from build123d import *

# Parameters (mm, degrees)
ESQUISSE1_R             = 15
BOSS_EXTRU_1_DEPTH      = 10
ESQUISSE2_R             = 12.5
BOSS_EXTRU_2_DEPTH      = 1
ESQUISSE3_R             = 11
ENL_V_MAT_EXTRU_1_DEPTH = 2
ESQUISSE4_R             = 12.5
ENL_V_MAT_EXTRU_2_DEPTH = 9


with BuildPart() as part:
    # Esquisse1 → Boss.-Extru.1 (new body)
    with BuildSketch(Plane.XY):
        Circle(ESQUISSE1_R)
    extrude(amount=BOSS_EXTRU_1_DEPTH)

    # Esquisse2 → Boss.-Extru.2 (add)
    with BuildSketch(Plane.XY.offset(10)):
        Circle(ESQUISSE2_R)
    extrude(amount=BOSS_EXTRU_2_DEPTH)

    # Esquisse3 → Enlèv. mat.-Extru.1 (cut)
    with BuildSketch(Plane.XY.offset(11)):
        Circle(ESQUISSE3_R)
    extrude(amount=-ENL_V_MAT_EXTRU_1_DEPTH, mode=Mode.SUBTRACT)

    # Esquisse4 → Enlèv. mat.-Extru.2 (cut)
    with BuildSketch(Plane(origin=(0, 0, 0), x_dir=(-1, 0, 0), z_dir=(0, 0, -1))):
        with Locations(Location((0, 0, 0), (0, 0, 180))):
            Circle(ESQUISSE4_R)
    extrude(amount=-ENL_V_MAT_EXTRU_2_DEPTH, mode=Mode.SUBTRACT)


solid = part.part
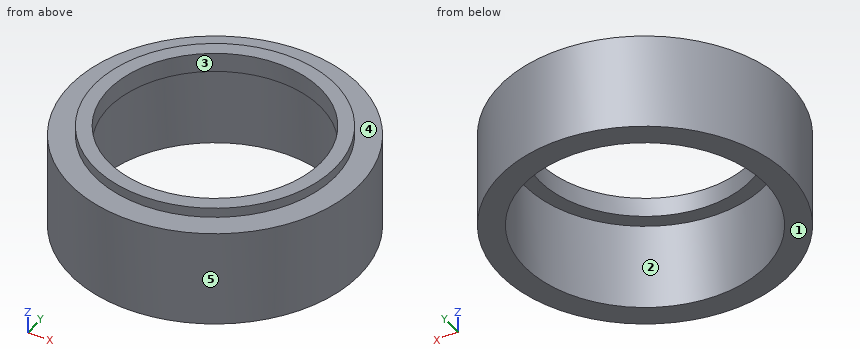
Input: part model. Units: mm. Frame: model coordinates. Face numbers are marked on the shaded views. A direction names the side the tool comes from. Give positions to 0.01 mm unless a question says otherwise; leave off trailing zeros. Order: outer loops, then holes, each group sorted by start corner. A loop starts at its lowest first (then second) coordinate and runs counter-clockwise, first axis right, second up. Notation, with made-up numbers: (53, -38) - (68, -38) arc R6 cw to (68, -29) - close; hole circle Ø7 at (-13, 73). An arc over 180 degrees is marked (long way). Write each question's results on one line, items separated by ' | '.
Item 1: Draft query along X for the marked faces 3, 4 and 5. Return one class per face: released by +X, released by -X, zero draft, split by the parting line, or undercut.
A:
face 3: undercut | face 4: zero draft | face 5: split by the parting line
Item 2: Contact query for flat-ended pins moving along their axis: pin 1 Ø17.5 at (x, y) = (0, 0) entering from -Z; pin 2 Ø5 at (y, z) = (-10, 8) entering from -X; pin 3 Ø5 at (y, z) = (-11.5, 2.5) entering from +X; pin 4 Ø2 at (y, z) = (-8, 6) entering from -X. Output: stop coordinate, or through.
A:
pin 1: passes through | pin 2: stops at x = -12.99 | pin 3: stops at x = 12 | pin 4: stops at x = -13.27
Item 3: Section D-D (x = 11.5). Return loops of the section in (y, z), and give its area (3 significant figures).
A:
outline: (-9.63, 0) - (-4.9, 0) - (-4.9, 9) - (4.9, 9) - (4.9, 0) - (9.63, 0) - (9.63, 10) - (4.9, 10) - (4.9, 11) - (-4.9, 11) - (-4.9, 10) - (-9.63, 10) - close | area: 114 mm^2
Item 4: Section C-C (z = 1.75). Return loops of the section in (x, y), and give its area (3 significant figures).
A:
outline: circle Ø30 at (0, 0); hole circle Ø25 at (0, 0) | area: 216 mm^2
Item 5: Access query for the marked faces 1 and 2. Directions: +Z, -Z, +X, -X, +Y, -Y. A direction counts if a zero-diameter tool reaches every point of the face in a straight line with its end or side. Return the directions, or none.
A:
face 1: -Z, +X, -X, +Y, -Y | face 2: -Z
Item 6: Material intervals for line 1 along X through (y, z) = (-0.25, 4.75); line 2 along Y through (x, z) = (0, 10.3); line 3 along Y through (x, z) = (0, 9.5), sorted ascending.
A:
line 1: x = -15 to -12.5, 12.5 to 15 | line 2: y = -12.5 to -11, 11 to 12.5 | line 3: y = -15 to -11, 11 to 15
Item 7: Section A-A (y = 0). Return loops of the section in (x, z).
A:
outline: (-15, 0) - (-12.5, 0) - (-12.5, 9) - (-11, 9) - (-11, 11) - (-12.5, 11) - (-12.5, 10) - (-15, 10) - close; (11, 9) - (12.5, 9) - (12.5, 0) - (15, 0) - (15, 10) - (12.5, 10) - (12.5, 11) - (11, 11) - close
